Study the drawing (mm; zero at the part's minimum x, y, z) and answer. A direction names the side the tool comes from. Give positions to 0.01 mm unless a question says otherwise; leave off trailing zeros. Write each loop counter-clockwise with the first axis right and the second up, starting at its lowest first coordinate (ties: lowest second). Pieces come first, ordered by that corner, then holes. Notation, with made-up numbers: M 77,56 L 126,56 A13 cw 126,81 Z; hole C 31,-4 d6. An arc over 180 degrees is marked long. Use a Markdown table: item, result. Add a question column.
Item 1: For the marked faces 1 and 2, determine the directions among +Z, -Z, +X, -X, +Y, -Y from which every point of the face is accessible in a straight line to the end or side of a thin tool.
Item 2: Given P1, Ø1, axis at y = 83.5, z = 88, coming from the +X side; P2, Ø0.5, axis at y = 103.5, z = 86.5, coming from the -X side; P3, Ø1.5, axis at x = 107, z = 63.5, coming from the +Y side, each flat-ended and moving along its own axis, determine where each tip first touches the part or whether it passes through.
Item 3: A cutting plane is placed at A-A on z = 28. Determine the outline of the cut face in (x, y).
Item 4: Consider probe 1 along Z at (x, y) = (2.5, 82); probe 2 along X at (y, z) = (61, 87.5); probe 3 along X at (y, z) = (56, 27.5). Determine where each line is inside the solid, lowest interval first. Write a range as [from, to].
Item 5: A cutting plane is placed at D-D on y = 24.5. Determine the outline of the cut face in (x, z), then the cut area to 3 significant figures.
Item 6: A cutting plane is placed at B-B on x = 2.5. Determine the outline of the cut face in (y, z), then the cut area to 3 significant figures.
Item 7: A cutting plane is placed at C-C on z = 87.5. Determine the outline of the cut face in (x, y), then the cut area to 3 significant figures.
Item 8: The mould has two halves that part along Z. Classify the marked faces 3, 4, 5 and 6: pulls with the +Z half, pulls with the -Z half, needs draft (parallel to the pull), parting line crosses it, or undercut.
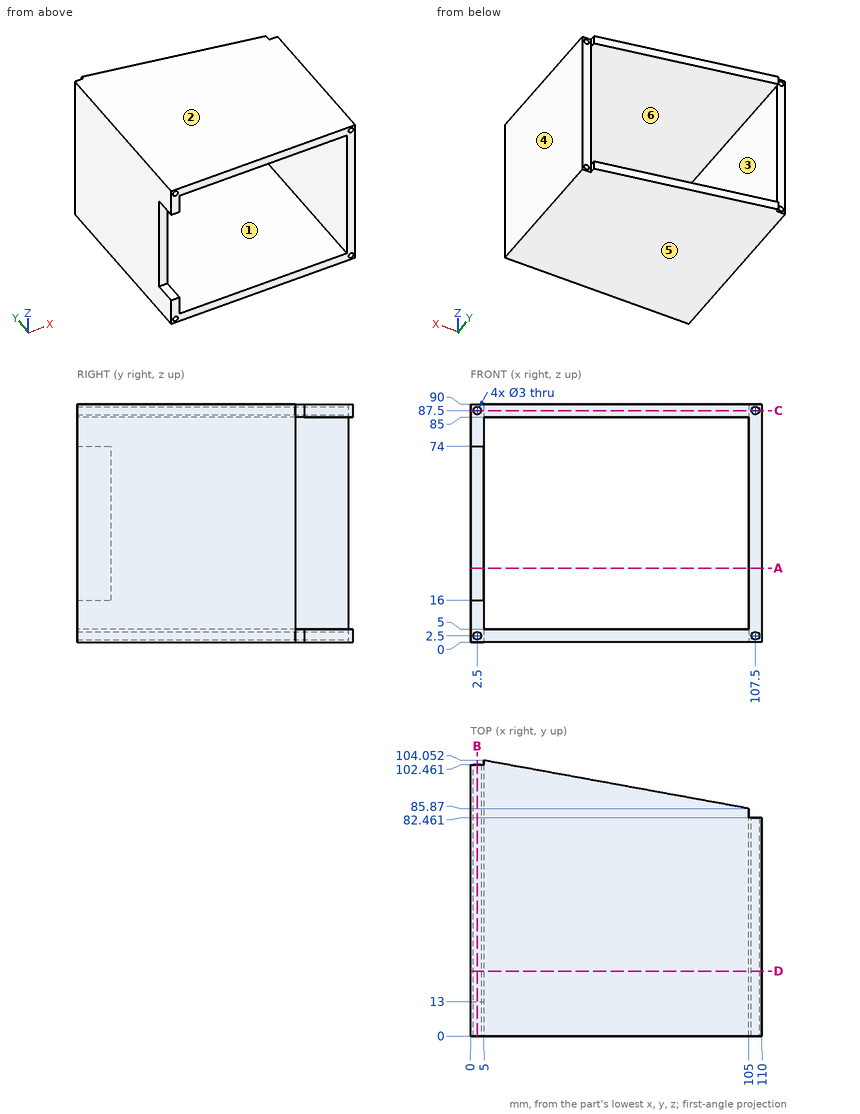
Filled in:
| question | item | result |
|---|---|---|
| 1 | face 1 | +Y, -Y |
| 1 | face 2 | +Z, +X, -X, +Y, -Y |
| 2 | P1 | x = 105 |
| 2 | P2 | x = 5 |
| 2 | P3 | y = 82.46 |
| 3 | outline | M 0,13 L 5,13 L 5,102.46 L 0,102.46 Z; M 105,0 L 110,0 L 110,82.46 L 105,82.46 Z |
| 4 | probe 1 | [0, 1], [4, 86], [89, 90] |
| 4 | probe 2 | [0, 1], [4, 106], [109, 110] |
| 4 | probe 3 | [0, 5], [105, 110] |
| 5 | outline | M 0,0 L 110,0 L 110,90 L 0,90 Z; hole C 2.5,2.5 d3; hole C 2.5,87.5 d3; hole M 5,5 L 105,5 L 105,85 L 5,85 Z; hole C 107.5,2.5 d3; hole C 107.5,87.5 d3 |
| 5 | area | 1,870 mm² |
| 6 | outline | M 0,0 L 102.46,0 L 102.46,1 L 0,1 Z; M 0,4 L 102.46,4 L 102.46,86 L 0,86 L 0,74 L 13,74 L 13,16 L 0,16 Z; M 0,89 L 102.46,89 L 102.46,90 L 0,90 Z |
| 6 | area | 7,850 mm² |
| 7 | outline | M 0,0 L 1,0 L 1,102.46 L 0,102.46 Z; M 4,0 L 106,0 L 106,82.46 L 105,82.46 L 105,85.87 L 5,104.05 L 5,102.46 L 4,102.46 Z; M 109,0 L 110,0 L 110,82.46 L 109,82.46 Z |
| 7 | area | 9,870 mm² |
| 8 | face 3 | undercut |
| 8 | face 4 | needs draft |
| 8 | face 5 | pulls with the -Z half |
| 8 | face 6 | undercut |
